Autodesk Inventor part; units mm, degrees
ref_plane "YZ Plane" through (0, 0, 0) normal (1, 0, 0) x (0, 1, 0)
ref_plane "XZ Plane" through (0, 0, 0) normal (0, 1, 0) x (-1, 0, 0)
sketch "Sketch1" plane through (0, 0, 0) normal (0, 0, 1) x (1, 0, 0)
  line L0 (0, 0) -> (8, 0)
  line L1 (8, 0) -> (8, 11)
  line L2 (8, 11) -> (0, 11)
  line L3 (0, 11) -> (0, 0)
  dimension "d0" = 8
  dimension "d1" = 11
extrude "Extrusion1" add sketch "Sketch1" along normal blind 5
sketch "Sketch2" plane through (0, 0, 5) normal (0, 0, 1) x (1, 0, 0)
  circle A0 centre (4, 7.251) radius 2.4
  circle A1 centre (4, 2.176) radius 1.575
  line L0 (4, 10.5689) -> (4, 1.2689) construction
  line L1 (0, 11) -> (0, 0)
  line L2 (8, 0) -> (8, 11)
  dimension "d4" = 3.15
  dimension "d5" = 4.8
  dimension "d6" = 1.1
  dimension "d7" = 4
  dimension "d8" = 4
extrude "Extrusion2" cut sketch "Sketch2" against normal blind 7
sketch "Sketch4" plane through (0, 0, 5) normal (0, 0, 1) x (1, 0, 0)
  line L0 (0, 0) -> (8, 0)
  line L1 (8, 0) -> (8, 4.2)
  line L2 (8, 4.2) -> (0, 4.2)
  line L3 (0, 4.2) -> (0, 0)
  line L4 (8, 0) -> (8, 11)
  circle A0 centre (4, 7.251) radius 2.4
  circle A1 centre (4, 2.176) radius 1.575
  dimension "d14" = 4.2
extrude "Extrusion4" cut sketch "Sketch4" against normal blind 2 contours L3 L2 L1 L0
fillet "Rundung1" radius 1 4 edges at (0, 11, 2.5) (8, 11, 2.5) (0, 4.2, 4) (8, 4.2, 4)
chamfer "Fase1" distance 0.5 angle 45 5 edges at (8, 5, 0) (7.7071, 10.7071, 0) (4, 11, 0) (0.2929, 10.7071, 0) (0, 5, 0)
properties part number "holder_test"
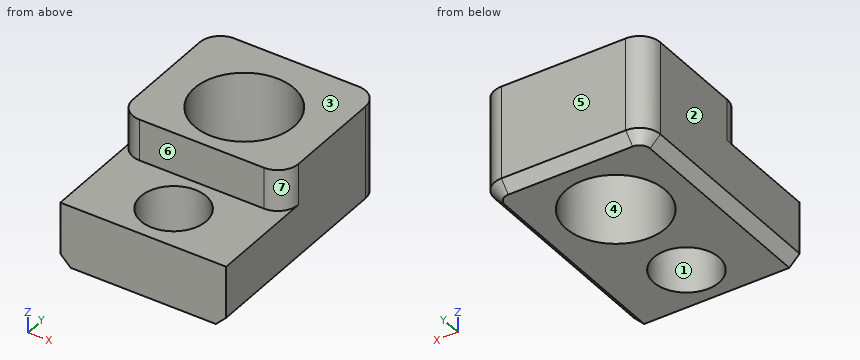
Build history of the part. All positions in model axes, mm. Face numbers are marked on the shaded views. A direction names the side the tool comes from. Give positions to 0.01 mm unless a question says otherwise; leave off trailing zeros. Write each loop counter-clockwise with the first axis right and the second up, starting at its lowest first coordinate (ties: lowest second). Pieces come first, ordered by that corner, then holes. Notation, with made-up numbers: (1, 80.5) - (45, 80.5) arc R10 ccw to (45, 95.5) - close; hole circle Ø10 at (72, 77). An arc over 180 degrees is marked (long way). Use one line per item in the form item = value. Start each with the question number.
1. Probe line 1 (Y direction, x = 4, z = 1.4); line 2 (Y direction, x = 4.75, z = 2.6); line 3 (Z direction, x = 1.5, y = 3.75). List the from-to ranges inside material, lowest first. Write a range as [from, to].
2. Two-plate mould, pull along X, no slides. Class the marked faces 1, 2, 3 and 4: released by +X, released by -X, zero draft, split by the parting line, or undercut.
3. Band-saw the part on C-C on z = 4.65. Write the cut outline in (x, y).
4. Band-saw the part on D-D on x = 1.75. Write the cut outline in (y, z).
5. 3-axis set-ups, long thin cutter, end or side, ignore diameter. For the marked faces 5, 6 and 7: which of +Z, -Z, +X, -X, +Y, -Y reach the whole face in a straight line?
6. Drop a flat-ended pin along its axis: pin 1 Ø1 at (x, z) = (3, 4) entering from -Y. Give the stop position or say it passes through.
7. Band-saw the part on A-A on x = 4. Write the cut outline in (y, z), plus the area to 3 significant figures.
8. Band-saw the part on B-B on y = 3.25. Write the cut outline in (x, z), plus the area to 3 significant figures.
Conclusion:
q1.line_1 = [0, 0.6], [3.75, 4.85], [9.65, 11]
q1.line_2 = [0, 0.79], [3.56, 4.97], [9.53, 11]
q1.line_3 = [0, 3]
q2.face_1 = undercut
q2.face_2 = released by -X
q2.face_3 = zero draft
q2.face_4 = undercut
q3.outline = (0, 5.2) arc R1 ccw to (1, 4.2) - (7, 4.2) arc R1 ccw to (8, 5.2) - (8, 10) arc R1 ccw to (7, 11) - (1, 11) arc R1 ccw to (0, 10) - close; hole circle Ø4.8 at (4, 7.25)
q4.outline = (0, 0) - (6.42, 0) - (6.42, 5) - (4.2, 5) - (4.2, 3) - (0, 3) - close; (8.09, 0) - (10.5, 0) - (11, 0.5) - (11, 5) - (8.09, 5) - close
q5.face_5 = +Z, -Z, +X, -X, +Y
q5.face_6 = +Z, +X, -X, -Y
q5.face_7 = +Z, +X, -Y
q6.pin_1 = 4.2
q7.outline = (0, 0) - (0.6, 0) - (0.6, 3) - (0, 3) - close; (3.75, 0) - (4.85, 0) - (4.85, 5) - (4.2, 5) - (4.2, 3) - (3.75, 3) - close; (9.65, 0) - (10.5, 0) - (11, 0.5) - (11, 5) - (9.65, 5) - close
q7.area = 13.0 mm²
q8.outline = (0, 0.5) - (0.5, 0) - (2.85, 0) - (2.85, 3) - (0, 3) - close; (5.15, 0) - (7.5, 0) - (8, 0.5) - (8, 3) - (5.15, 3) - close
q8.area = 16.8 mm²
